Source: CAD feature listing. Evaluate the final solid. Frame: model axes, mm. A direction names the side the tool comes from. Round coordinates to 2 decimals unless told otherwise and drop trailing zeros. Loops run counter-clockwise (first coordinate to the right, second up) from the corner with the lowest first, then second, coordinate; pieces in that order, holes last. Notation, with made-up numbers: M 0.5,29 L 4.5,29 A26 cw 4.5,45 Z; hole C 65.25,3 d5. An arc over 180 degrees is marked long. Answer as a JSON object with one key per item and string values.
Autodesk Inventor part; units mm, degrees
ref_plane "Work Plane1" through (0, 4, 0) normal (0, 1, 0) x (-1, 0, 0)
ref_plane "YZ Plane" through (0, 0, 0) normal (1, 0, 0) x (0, 1, 0)
ref_plane "XY Plane" through (0, 0, 0) normal (0, 0, 1) x (1, 0, 0)
sketch "Sketch1" plane through (0, 0, 0) normal (0, 0, 1) x (1, 0, 0)
  circle A0 centre (0, 0) radius 4
  dimension "d0" = 8
extrude "Extrusion1" add sketch "Sketch1" along normal mid plane 55
chamfer "Chamfer1" distance 0.5 angle 45 2 edges at (-4, 0, 27.5) (-4, 0, -27.5)
ref_plane "Work Plane1" through (0, 4, 0) normal (0, 1, 0) x (-1, 0, 0)
sketch "Sketch2" plane through (0, 4, 0) normal (0, 1, 0) x (-1, 0, 0)
  line L0 (-3.5, 27.5) -> (3.5, 27.5)
  line L1 (4, -27) -> (4, 27)
  line L2 (1, 19.5) -> (-1, 19.5)
  line L3 (-1, 19.5) -> (-1, 10.5)
  line L4 (-1, 10.5) -> (1, 10.5)
  line L5 (1, 10.5) -> (1, 19.5)
  point P0 (0, 0)
  dimension "d7" = 2
  dimension "d8" = 9
  dimension "d9" = 8
  dimension "d10" = 1
extrude "Extrusion2" cut sketch "Sketch2" against normal blind 2
fillet "Fillet1" radius 0.1 4 edges at (1, 3.873, 15) (0, 4, 10.5) (-1, 3.873, 15) (0, 4, 19.5)
properties part number "asGearbox" material "Stainless Steel"
Item 1: Contact query for flat-ended pins moving along their axis: pin 1 Ø2 at (x, z) = (2.5, -10) entering from +Y; pin 2 Ø1.4 at (y, z) = (2.5, 13) entering from -X; pin 3 Ø0.9 at (y, z) = (2.5, 17) entering from +X. Output: stop coordinate, or through.
Answer sheet:
{"pin 1": "stops at y = 3.71", "pin 2": "stops at x = -3.57", "pin 3": "stops at x = 3.43"}
Item 2: Access query for faces 1 (the flat face through (0, 2, 15)), 2 (the cylindrical face through (2.15, -3.373, -0.378)). Directions: +Z, -Z, +X, -X, +Y, -Y. A direction counts if a zero-diameter tool reaches every point of the face in a straight line with its end or side. Return the directions, or none.
Answer sheet:
{"face 1": "+Y", "face 2": "+Z, -Z"}
Item 3: Pull-direction query (Z, two-part tool) for faces 3 (the flat face through (1, 3, 15)), 4 (the flat face through (0, 0, 27.5)), 5 (the flat face through (0, 3, 10.5)), 6 (the flat face through (0, 0, -27.5)); classes: pulls with the +Z half, pulls with the -Z half, needs draft (parallel to the pull), parting line crosses it, or undercut.
Answer sheet:
{"face 3": "undercut", "face 4": "pulls with the +Z half", "face 5": "undercut", "face 6": "pulls with the -Z half"}
Item 4: Line query: probe 1 along Y at (x, z) = (0.25, 9); probe 2 along Y at (x, z) = (0.25, 15); probe 3 along X at (y, z) = (-3, 24). Output: solid intervals per line, ascending. Write a range as from..to.
Answer sheet:
{"probe 1": "y = -3.99..3.99", "probe 2": "y = -3.99..2", "probe 3": "x = -2.65..2.65"}
Item 5: Section A-A on x = 0. Return the cut outline in (y, z), then the cut area to 3 significant figures.
Answer sheet:
{"outline": "M -4,-27 L -3.5,-27.5 L 3.5,-27.5 L 4,-27 L 4,10.4 A0.1 ccw 3.9,10.5 L 2,10.5 L 2,19.5 L 3.9,19.5 A0.1 ccw 4,19.6 L 4,27 L 3.5,27.5 L -3.5,27.5 L -4,27 Z", "area": "421 mm²"}
Item 6: Section B-B on z = -20. Return the cut outline in (x, y), then the cut area to 3 significant figures.
Answer sheet:
{"outline": "C 0,0 d8", "area": "50.3 mm²"}
